from build123d import *

# Parameters (mm, degrees)
F0_W     = 38.1
F0_H     = 38.1
F1_DEPTH = 25.4
F2_R     = 1.5875
F3_DEPTH = 38.1
F4_R     = 12.7
F5_DEPTH = 25.4


with BuildPart() as f1:
    # F0 (on Top) → F1 (new body)
    with BuildSketch(Plane.XY):
        with Locations((19.05, 19.05)):
            Rectangle(F0_W, F0_H)
    extrude(amount=F1_DEPTH)

    # F2 (on face) → F3 (cut)
    with BuildSketch(Plane.YZ.offset(38.1)):
        with Locations((19.05, 12.7)):
            Circle(F2_R)
    extrude(amount=-F3_DEPTH, mode=Mode.SUBTRACT)

    # F4 (on face) → F5 (cut)
    with BuildSketch(Plane.XY.offset(25.4)):
        with Locations((19.05, 19.05)):
            Circle(F4_R)
    extrude(amount=-F5_DEPTH, mode=Mode.SUBTRACT)


solid = f1.part
Can you work these out from the model? Positions are in its coordinate system, mm. Round coordinates to 2 decimals unless told otherwise and drop trailing zeros. Write each loop counter-clockwise with the first axis right and the second up, starting at its lowest first coordinate (ties: lowest second). Pieces come first, ordered by that corner, then holes. Notation, with made-up numbers: M -31.5,47.5 L -10.5,47.5 A19 ccw -10.5,54.5 Z; hole C 8,47 d8. An arc over 180 degrees is marked long. Use a Markdown table: item, result.
Item 1: If I drill on line 1 along Y through (x, z) = (19.05, 7.75); line 2 along Y through (x, z) = (4.5, 12.7), over which ranges is the centre line in solid material (lowest first)? Write a range as [from, to].
Found:
| item | result |
|---|---|
| line 1 | y = [0, 6.35], [31.75, 38.1] |
| line 2 | y = [0, 17.46], [20.64, 38.1] |
Item 2: I want a section at C-C (x = 19.05). List the corners of the cut face in (y, z) for me.
Found:
| item | result |
|---|---|
| outline | M 0,0 L 6.35,0 L 6.35,25.4 L 0,25.4 Z; M 31.75,0 L 38.1,0 L 38.1,25.4 L 31.75,25.4 Z |
Item 3: We'd pull the mould along Y, two halves only. Please class faces 1 (the face through (0, 19, 15)), 2 (the face through (34.92, 17.88, 13.773)), 3 (the face through (19, 0, 13)): released by +Y, released by -Y, zero draft, split by the parting line, or undercut.
Found:
| item | result |
|---|---|
| face 1 | zero draft |
| face 2 | undercut |
| face 3 | released by -Y |
Item 4: I want a section at B-B (z = 12.7). List the corners of the cut face in (x, y) for me.
Found:
| item | result |
|---|---|
| outline | M 0,0 L 38.1,0 L 38.1,17.46 L 31.65,17.46 A12.7 cw 6.45,17.46 L 0,17.46 Z; M 0,20.64 L 6.45,20.64 A12.7 cw 31.65,20.64 L 38.1,20.64 L 38.1,38.1 L 0,38.1 Z |
Item 5: I want a section at D-D (y = 25.5). List the corners of the cut face in (x, z) for me, and give its area (3 significant figures).
Found:
| item | result |
|---|---|
| outline | M 0,0 L 8.11,0 L 8.11,25.4 L 0,25.4 Z; M 29.99,0 L 38.1,0 L 38.1,25.4 L 29.99,25.4 Z |
| area | 412 mm2 |
Item 6: I want a section at A-A (y = 19.05). List the corners of the cut face in (x, z) for me.
Found:
| item | result |
|---|---|
| outline | M 0,0 L 6.35,0 L 6.35,11.11 L 0,11.11 Z; M 0,14.29 L 6.35,14.29 L 6.35,25.4 L 0,25.4 Z; M 31.75,0 L 38.1,0 L 38.1,11.11 L 31.75,11.11 Z; M 31.75,14.29 L 38.1,14.29 L 38.1,25.4 L 31.75,25.4 Z |
